Design review of the part shown in the three views and the two pictorial views. Dimensions are in mm from the part's minimum x, y and z. A direction names the side the tool comes from. Coordinates: 2 decimals unless noted, no trailing zeros. Loops run counter-clockwise (first coordinate to the right, second up) from the corner with the lowest first, then second, coordinate; pieces in that order, holes last. Notation, with made-up numbers: M 12,-35 L 56,-35 A19 ccw 56,1 Z; hole C -2.5,73.5 d10. An arc over 180 degrees is marked long. Use one line per item in the form item = value.
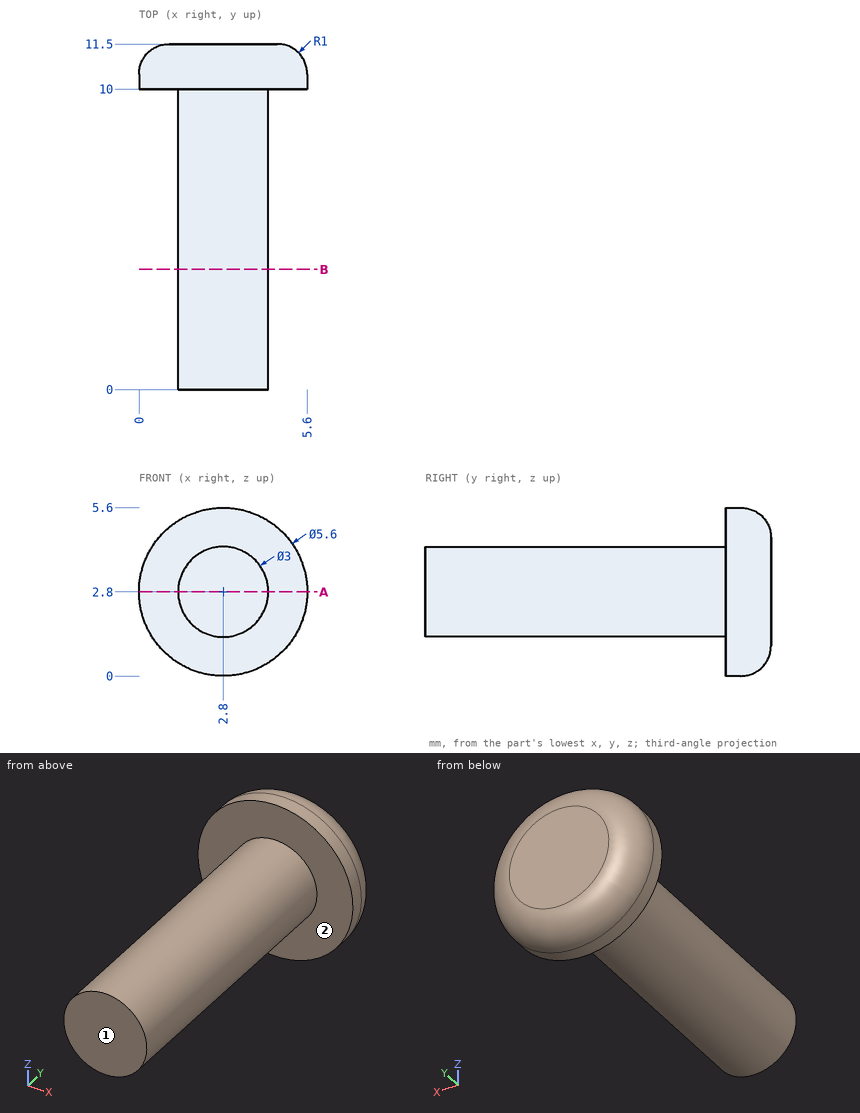
1. Machinability: for the marked faces 1 and 2, which of the approach directions +Z, -Z, +X, -X, +Y, -Y give a long, thin tool a straight path to every point of the face, cutting with its end or side? Answer none if there is none.
Response values:
face_1 = +Z, -Z, +X, -X, -Y
face_2 = -Y
2. Add section A-A (z = 2.8). State the section outline as (x, y) points, then the cut area to 3 significant figures.
Response values:
outline = M 0,10 L 1.3,10 L 1.3,0 L 4.3,0 L 4.3,10 L 5.6,10 L 5.6,10.5 A1 ccw 4.6,11.5 L 1,11.5 A1 ccw 0,10.5 Z
area = 38.0 mm^2
3. Wall thickness on line 1 along Y through (x, z) = (0.55, 1.7); line 2 along Z through (x, y) = (3.15, 6.75); line 3 along Y through (x, z) = (1.2, 1.75): over which ranges is each line inside the solid? List them lowest first. Write a range as from..to.
Response values:
line_1 = 10..11.21
line_2 = 1.34..4.26
line_3 = 10..11.49
4. Add section B-B (y = 4). State the section outline as (x, z) points, then the cut area to 3 significant figures.
Response values:
outline = C 2.8,2.8 d3
area = 7.07 mm^2
5. Insertion check: P1, Ø3, axis at y = 3.5, z = 3.5, coming from the +X side; P2, Ø2, axis at y = 8.5, z = 4, coming from the -X side; P3, Ø2, axis at y = 6, z = 5, coming from the -X side. Each pin has a flat end and moves straight along its axis. Give the tip position at first contact, or say it passes through.
Response values:
P1 = 4.3
P2 = 1.31
P3 = 1.9
